from build123d import *

# Parameters (mm, degrees)
SKETCH_1_R      = 3.25
SKETCH_1_R_2    = 6.5
SKETCH_1_R_3    = 1.6
EXTRUDE_2_DEPTH = 1.6


with BuildPart() as part:
    # 草图1 → 凸台-拉伸2 (new body)
    with BuildSketch(Plane.XY):
        with BuildLine():
            Line((-50, 20), (-41, 20))
            ThreePointArc((-41, 20), (-39.585786438, 19.414213562), (-39, 18))
            Line((-39, 18), (-39, -3))
            ThreePointArc((-39, -3), (-39.585786438, -4.414213562), (-41, -5))
            Line((-41, -5), (-50, -5))
            Line((-50, -5), (-50, -24.506949679))
            add(Edge.make_bspline(
                [(-50, -24.506949679), (-26.057041225, -37.751626241), (-24.673757374, -65)],
                knots=[0, 0, 0, 1, 1, 1], degree=2))
            Line((-24.673757374, -65), (24.673757374, -65))
            add(Edge.make_bspline(
                [(50, -24.506949679), (26.057041225, -37.751626241), (24.673757374, -65)],
                knots=[0, 0, 0, 1, 1, 1], degree=2))
            Line((50, -24.506949679), (50, -5))
            Line((50, -5), (41, -5))
            ThreePointArc((41, -5), (39.585786438, -4.414213562), (39, -3))
            Line((39, -3), (39, 18))
            ThreePointArc((39, 18), (39.585786438, 19.414213562), (41, 20))
            Line((41, 20), (50, 20))
            Line((50, 20), (50, 35))
            Line((50, 35), (3.25, 35))
            ThreePointArc((3.25, 35), (0, 31.75), (-3.25, 35))
            Line((-3.25, 35), (-50, 35))
            Line((-50, 35), (-50, 20))
        make_face()
        with Locations((0, -35)):
            Circle(SKETCH_1_R, mode=Mode.SUBTRACT)
        with Locations((30.310889132, -17.5)):
            Circle(SKETCH_1_R_2, mode=Mode.SUBTRACT)
        with Locations((30.310889132, 17.5)):
            Circle(SKETCH_1_R_2, mode=Mode.SUBTRACT)
        with Locations((-30.310889132, 17.5)):
            Circle(SKETCH_1_R_2, mode=Mode.SUBTRACT)
        with Locations((-30.310889132, -17.5)):
            Circle(SKETCH_1_R_2, mode=Mode.SUBTRACT)
        with Locations((0, -41.5)):
            Circle(SKETCH_1_R_3, mode=Mode.SUBTRACT)
    extrude(amount=EXTRUDE_2_DEPTH)


solid = part.part
The model under review builds one solid part; all positions refer to its coordinate system, in mm. Coordinates: 2 decimals unless noted, no trailing zeros. Write each loop counter-clockwise with the first axis right and the second up, starting at its lowest first coordinate (ties: lowest second). Pieces come first, ordered by that corner, then holes. Notation, with made-up numbers: (32, -30.5) -> (86, -30.5) arc R23 ccw to (86, -15.5) -> close; hole circle Ø2 at (87.5, 30). An arc over 180 degrees is marked (long way). Answer in a Markdown table with one row per item.
1. Wall thickness on probe 1 along X at (y, z) = (-17, 1); probe 2 along Y at (x, z) = (0, 1.35); probe 3 along X at (y, z) = (17, 0.1): over which ranges is each line inside the solid? List them lowest first. Write a range as [from, to].
Answers below:
| item | result |
|---|---|
| probe 1 | x = [-50, -36.79], [-23.83, 23.83], [36.79, 50] |
| probe 2 | y = [-65, -43.1], [-39.9, -38.25], [-31.75, 31.75] |
| probe 3 | x = [-39, -36.79], [-23.83, 23.83], [36.79, 39] |
2. We need section A-A, the plane x = 0. State the section outline as (y, z) points.
Answers below:
| item | result |
|---|---|
| outline | (-65, 0) -> (-43.1, 0) -> (-43.1, 1.6) -> (-65, 1.6) -> close; (-39.9, 0) -> (-38.25, 0) -> (-38.25, 1.6) -> (-39.9, 1.6) -> close; (-31.75, 0) -> (31.75, 0) -> (31.75, 1.6) -> (-31.75, 1.6) -> close |
3. We need section B-B, the plane y = -17.5. State the section outline as (x, z) points, and give its area (3 significant figures).
Answers below:
| item | result |
|---|---|
| outline | (-50, 0) -> (-36.81, 0) -> (-36.81, 1.6) -> (-50, 1.6) -> close; (-23.81, 0) -> (23.81, 0) -> (23.81, 1.6) -> (-23.81, 1.6) -> close; (36.81, 0) -> (50, 0) -> (50, 1.6) -> (36.81, 1.6) -> close |
| area | 118 mm^2 |
4. We need section C-C, the plane z = 0.55. Give the number of separate pieces and of enclosed holes in the cut face, and give its area (3 significant figures).
Answers below:
| item | result |
|---|---|
| separate pieces | 1 |
| enclosed holes | 6 |
| area | 7,420 mm^2 |
5. Draft analysis for pull direction Y (two halves, no side actions). For faces 1 (the cylindrical face through (36.51, 19.45, 0.79)), 2 (the cylindrical face through (-0.705, -38.173, 0.789)), 3 (the flat face through (-1, -14, 0)), 4 (the cylindrical face through (0.07, 31.75, 0.79)), state which applies: +Y half, -Y half, draft (parallel to the pull), parting line (faces both ways), or undercut.
Answers below:
| item | result |
|---|---|
| face 1 | undercut |
| face 2 | undercut |
| face 3 | draft |
| face 4 | +Y half |
